Input: part model. Units: mm. Frame: model coordinates. Face numbers are marked on the shaded views. A direction names the side the tool comes from. Give positions to 0.01 mm unless a question says otherwise; leave off trailing zeros. Loops run counter-clockwise (first coordinate to the right, second up) from the corner with the lowest first, then second, coordinate; pieces in that order, holes last. Notation, with made-up numbers: M -40,86 L -33,86 A14 cw -33,105 Z; hole C 65,-0.75 d11. An arc over 180 degrees is marked long. One line per item, written item: value. Start each with the question number.
(1) Pull-direction query (Y, two-part tool) for the marked faces 4, 5, 6 and 7; classes: released by +Y, released by -Y, zero draft, split by the parting line, or undercut.
(2) Pin query (flat end, axial travel): P1, Ø1.5, axis at x = 5.5, y = 0, coming from the -Z side; P2, Ø3, axis at x = -0.5, y = 2, coming from the +Z side. Return the tip coordinate at first contact, or that it passes through.
(3) Section B-B on x = 2. Output: boundary loops of the cut face in (y, z), plus the area to 3 significant figures.
(4) Section A-A on x = -1.25. Output: boundary loops of the cut face in (y, z).
(5) Ray query, line 1 along Y through (x, z) = (1.75, 0.1); line 2 along X through (y, z) = (1.45, 1.9). Return the intervals inside material, ascending. Write a range as from..to.
(6) Section C-C on z = 2.35. Output: boundary loops of the cut face in (x, y).
(7) Access query for the marked faces 1, 2 and 3. Directions: +Z, -Z, +X, -X, +Y, -Y. A direction counts if a zero-diameter tool reaches every point of the face in a straight line with its end or side. Return the directions, or none.
Autodesk Inventor part; units mm, degrees
ref_plane "YZ Plane" through (0, 0, 0) normal (1, 0, 0) x (0, 1, 0)
ref_plane "XZ Plane" through (0, 0, 0) normal (0, 1, 0) x (-1, 0, 0)
ref_plane "XY Plane" through (0, 0, 0) normal (0, 0, 1) x (1, 0, 0)
sketch "Sketch_1" plane through (0, 0, 0) normal (0, 0, 1) x (1, 0, 0)
  line L0 (8, 0) -> (-0.2321, 0)
  line L1 (-0.2321, 0) -> (-0.5, 1)
  line L2 (-0.5, 1) -> (-2, 1)
  line L3 (-2, 1) -> (-2, 2.75)
  line L4 (-2, 2.75) -> (0, 2.75)
  line L5 (0, 2.75) -> (0, 1.6)
  arc A0 (0, 1.6) -> (0.1, 1.5) centre (0.1, 1.6) ccw
  line L6 (0.1, 1.5) -> (7.6935, 1.5)
  line L7 (7.6935, 1.5) -> (8, 1.1935)
  line L8 (8, 1.1935) -> (8, 0)
  line L9 (8, 0) -> (-0.2321, 0)
revolve "Revolution1" add sketch "Sketch_1" angle 360 about axis through (8, 0, 0) along (1, 0, 0)
thread "Thread1"
sketch "Sketch_2" plane through (-2, 0, 0) normal (1, 0, 0) x (0, 0, -1)
  line L0 (-1, -0.5774) -> (0, -1.1547)
  line L1 (0, -1.1547) -> (1, -0.5774)
  line L2 (1, -0.5774) -> (1, 0.5774)
  line L3 (1, 0.5774) -> (0, 1.1547)
  line L4 (0, 1.1547) -> (-1, 0.5774)
  line L5 (-1, 0.5774) -> (-1, -0.5774)
extrude "Extrusion1" cut sketch "Sketch_2" along normal blind 1.5
properties part number "CBSH3-8" material "鋼"
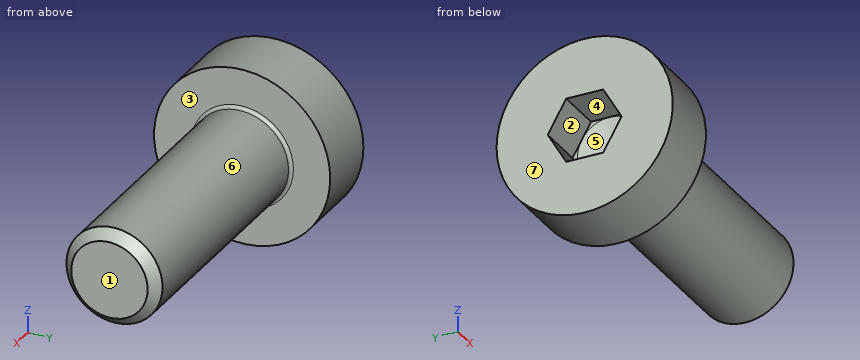
Output values:
1. face 4: undercut
1. face 5: undercut
1. face 6: split by the parting line
1. face 7: zero draft
2. P1: stops at z = -1.5
2. P2: stops at z = 2.7
3. outline: C 0,0 d3
3. area: 7.07 mm²
4. outline: C 0,0 d5.5; hole M -1.15,0 L -0.58,-1 L 0.58,-1 L 1.15,0 L 0.58,1 L -0.58,1 Z
5. line 1: y = -1.5..1.5
5. line 2: x = -2..0
6. outline: M -2,-1.43 L 0,-1.43 L 0,1.43 L -2,1.43 Z
7. face 1: +Z, -Z, +X, +Y, -Y
7. face 2: -X
7. face 3: +X
